Autodesk Inventor part; units mm, degrees
ref_plane "YZ Plane" through (0, 0, 0) normal (1, 0, 0) x (0, 1, 0)
ref_plane "XZ Plane" through (0, 0, 0) normal (0, 1, 0) x (-1, 0, 0)
ref_plane "XY Plane" through (0, 0, 0) normal (0, 0, 1) x (1, 0, 0)
sketch "Sketch1" plane through (0, 0, 0) normal (0, 1, 0) x (-1, 0, 0)
  line L0 (0, 0) -> (152.4, 0)
  line L1 (152.4, 0) -> (152.4, -68.58)
  line L2 (152.4, -68.58) -> (0, -68.58)
  line L3 (0, -68.58) -> (0, 0)
  dimension "d0" = 152.4
  dimension "d1" = 68.58
extrude "Extrusion1" add sketch "Sketch1" along normal blind 6.35
sketch "Sketch2" plane through (0, 6.35, 0) normal (0, 1, 0) x (1, 0, 0)
  line L0 (-133.35, 0) -> (-139.7, 0)
  line L1 (-139.7, 0) -> (-139.7, -12.7)
  line L2 (-139.7, -12.7) -> (-133.35, -12.7)
  line L3 (-133.35, -12.7) -> (-133.35, 0)
  circle A0 centre (-136.525, -9.525) radius 1.397
  line L4 (-152.4, 0) -> (0, 0)
  line L5 (-12.7, 0) -> (-19.05, 0)
  line L6 (-19.05, 0) -> (-19.05, -12.7)
  line L7 (-19.05, -12.7) -> (-12.7, -12.7)
  line L8 (-12.7, -12.7) -> (-12.7, 0)
  circle A1 centre (-15.875, -9.525) radius 1.397
  dimension "d4" = 12.7
  dimension "d5" = 6.35
  dimension "d6" = 2.794
  dimension "d7" = 3.175
  dimension "d8" = 3.175
  dimension "d9" = 0
  dimension "d10" = 12.7
  dimension "d11" = 12.7
  dimension "d12" = 6.35
  dimension "d13" = 2.794
  dimension "d14" = 3.175
  dimension "d15" = 3.175
  dimension "d16" = 0
  dimension "d17" = 12.7
extrude "Extrusion2" add sketch "Sketch2" against normal blind 6.35
ref_plane "Work Plane1" through (-133.35, 0, -34.29) normal (0, 0, 1) x (1, 0, 0)
mirror "Mirror1" about plane through (-133.35, 0, -34.29) normal (0, 0, 1) of "Extrusion2"
properties part number "BottomPanel"
Verification items for the finished model (mm, model axes). A direction names the side the tool comes from. Coordinates: 2 decimals unless noted, no trailing zeros. Order: outer loops, then holes, each group sorted by start corner. A loop starts at its lowest first (then second) coordinate and runs counter-clockwise, first axis right, second up. Notation, with made-up numbers: M 23.5,-36 L 71.5,-36 A12 cw 71.5,-22 Z; hole C 67,49.25 d1. An arc over 180 degrees is marked long. One line per item, written item: value. Start each with the question number.
Item 1: Access from +Z, -Z, +X, -X, +Y, -Y to the whole of each face (thin tool, end or side, straight path). Record for faces 4 (the flat face through (-6, 3, -68.58)), 5 (the flat face through (-146, 3, 0)), 6 (the flat face through (-139.7, 3, -75)), 7 (the flat face through (-133.35, 3, 6)).
Item 2: Mould release check, pull along X, two halves, no side actions. Record for faces 1 (the flat face through (-16, 3, -81.28)), 2 (the flat face through (-152.4, 3, -34)), 3 (the flat face through (-19.05, 3, -75)): pulls with the +X half, pulls with the -X half, needs draft (parallel to the pull), parting line crosses it, or undercut.
Item 3: Sectioned sample at A-A on z = -73.5. Record the cut outline in (x, y).
Item 4: Thickness scan on probe 1 along X at (y, z) = (1.5, -73.5); probe 2 along Z at (x, y) = (-68, 2.75). Record the ranges inside material, lowest first.
Item 5: Sectioned sample at C-C on x = -131. Record the cut outline in (y, z), then the cut area to 3 significant figures.
Item 6: Depth check by flat-ended pin: P1, Ø1.9, axis at y = 4, z = -72.5, coming from the +X side; P2, Ø3, axis at x = -92.5, y = 2, coming from the +Z side; P3, Ø1.9, axis at y = 3.5, z = 7.5, coming from the -X side; P4, Ø1.7, axis at x = -136.525, z = -78.105, coming from the -Y side. Enter the tip coordinate at first touch or a pass-through.
Item 7: Sectioned sample at B-B on y = 4.5. Record the cut outline in (x, z) (3 decimals), then the cut area to 3 significant figures.
Calculated:
1. face 4: -Z, +X, +Y, -Y
1. face 5: +Z, -X, +Y, -Y
1. face 6: -Z, -X, +Y, -Y
1. face 7: +Z, +Y, -Y
2. face 1: needs draft
2. face 2: pulls with the -X half
2. face 3: undercut
3. outline: M -139.7,0 L -133.35,0 L -133.35,6.35 L -139.7,6.35 Z; M -19.05,0 L -12.7,0 L -12.7,6.35 L -19.05,6.35 Z
4. probe 1: -139.7 to -133.35, -19.05 to -12.7
4. probe 2: -68.58 to 0
5. outline: M 0,-68.58 L 6.35,-68.58 L 6.35,0 L 0,0 Z
5. area: 435 mm^2
6. P1: x = -12.7
6. P2: z = 0
6. P3: x = -139.7
6. P4: through
7. outline: M -152.4,-68.58 L -139.7,-68.58 L -139.7,-81.28 L -133.35,-81.28 L -133.35,-68.58 L -19.05,-68.58 L -19.05,-81.28 L -12.7,-81.28 L -12.7,-68.58 L 0,-68.58 L 0,0 L -12.7,0 L -12.7,12.7 L -19.05,12.7 L -19.05,0 L -133.35,0 L -133.35,12.7 L -139.7,12.7 L -139.7,0 L -152.4,0 Z; hole C -136.525,-78.105 d2.794; hole C -136.525,9.525 d2.794; hole C -15.875,-78.105 d2.794; hole C -15.875,9.525 d2.794
7. area: 10,700 mm^2
